Can you work these out from the model? Positions are in its coordinate system, mm. A direction names the side the tool comes from. Coordinates: 2 decimals unless noted, no trailing zeros. Order: outer loops, then holes, each group sorted by start corner. A loop starts at its lowest first (then second) coordinate and runs counter-clockwise, first axis right, second up. Notation, with made-up numbers: (50, -6.75) -> (77, -6.75) arc R29 ccw to (77, 20.25) -> close; hole circle Ø2 at (78.5, 27). An arc over 180 degrees is marked (long way). Answer as a JSON object with one key per item and string values. Group by question number.
(1) Which directions (+Z, -Z, +X, -X, +Y, -Y) give clear straight access to the entire face, cutting with the end or side of a thin tool? Please do faces 4 (the flat face through (31.5, -30, 0)), 5 (the flat face through (33, -29, 0)), 6 (the flat face through (-49, -59.5, 0)), 7 (the flat face through (-33, -29, 0)).
(2) I need wall thicknesses on line 1 (X direction, y = -59.1, z = 0); line 2 (X direction, y = -34.5, z = 6.5); line 3 (X direction, y = -58.45, z = 0). Which ranges of each line are inside material? Lowest first, please.
(3) I want a section at C-C, the plane z = 0. List the corners of the cut face in (x, y) for me, plus the area to 3 significant figures.
(4) For pin 1 (11.5 mm diameter, centred on x = 59, z = 0, fed in from +Y); pin 2 (20 mm diameter, centred on y = -29, z = 8.5, fed in from -X); pin 3 (20 mm diameter, centred on y = -35.5, z = -4, fed in from +X), each with a flat end and sliding along its axis, tell me the tip position at first contact or that it passes through.
(5) I want a section at D-D, the plane x = -43.5. List the corners of the cut face in (y, z) for me.
(6) I want a section at A-A, the plane x = 64.5. List the corners of the cut face in (y, z) for me.
(7) I want a section at B-B, the plane y = -17. List the corners of the cut face in (x, z) for me, plus the area to 3 significant figures.
(8) If we mould it in two halves opening along Z, with no side actions, what happens to faces 1 (the flat face through (70, -59, 18)), 2 (the cylindrical face through (61.57, -58.74, -0.65)), 3 (the flat face through (-50, -58, 0))? For each: pulls with the +Z half, pulls with the -Z half, needs draft (parallel to the pull), parting line crosses it, or undercut.
from build123d import *

# Parameters (mm, degrees)
SKETCH1_W          = 60
SKETCH1_H          = 40
BASE_FLANGE1_DEPTH = 1.5
EDGE_FLANGE1_DEPTH = 40
EDGE_FLANGE2_DEPTH = 40
CHAMFER1_SIZE      = 5
CUT_EXTRUDE1_REACH = 97.357
SKETCH10_R         = 2
SKETCH10_R_2       = 3


# Sheet-metal steps are written as plain solids
with BuildPart() as part:
    # Sketch1 → Base-Flange1 (new body)
    with BuildSketch(Plane(origin=(0, 0, 0), x_dir=(1, 0, 0), z_dir=(0, 1, 0))):
        Rectangle(SKETCH1_W, SKETCH1_H)
    extrude(amount=-BASE_FLANGE1_DEPTH)

    # Edge-Flange1 section (across the edge) → Edge-Flange1 (add)
    with BuildSketch(Plane(origin=(-31.5, -1.5, 20), x_dir=(1, 0, 0), z_dir=(0, 0, -1))):
        with BuildLine():
            Line((-1.5, 1.5), (-1.5, 55))
            Line((-1.5, 55), (0, 55))
            Line((0, 55), (0, 1.5))
            ThreePointArc((0, 1.5), (0.439339828, 0.439339828), (1.5, 0))
            Line((1.5, 0), (1.5, -1.5))
            ThreePointArc((1.5, -1.5), (-0.621320344, -0.621320344), (-1.5, 1.5))
        make_face()
    edge_flange1 = extrude(amount=EDGE_FLANGE1_DEPTH)

    # Edge-Flange2 section (across the edge) → Edge-Flange2 (add)
    with BuildSketch(Plane(origin=(-33, -58, -20), x_dir=(0, 1, 0), z_dir=(0, 0, 1))):
        with BuildLine():
            Line((-1.5, 1.5), (-1.5, 40))
            Line((-1.5, 40), (0, 40))
            Line((0, 40), (0, 1.5))
            ThreePointArc((0, 1.5), (0.439339828, 0.439339828), (1.5, 0))
            Line((1.5, 0), (1.5, -1.5))
            ThreePointArc((1.5, -1.5), (-0.621320344, -0.621320344), (-1.5, 1.5))
        make_face()
    edge_flange2 = extrude(amount=EDGE_FLANGE2_DEPTH)

    # Mirror1: Edge-Flange1, Edge-Flange2 across plane
    add(edge_flange1.mirror(Plane(origin=(0, 0, 0), x_dir=(0, 0, 1), z_dir=(1, 0, 0))))
    add(edge_flange2.mirror(Plane(origin=(0, 0, 0), x_dir=(0, 0, 1), z_dir=(1, 0, 0))))

    # Chamfer1
    chamfer1_edges = [part.edges().sort_by_distance(p)[0] for p in [
        (-73, -58.75, -20),
        (-73, -58.75, 20),
        (73, -58.75, 20),
        (73, -58.75, -20),
    ]]
    chamfer(chamfer1_edges, length=CHAMFER1_SIZE)

    # Sketch10 → Cut-Extrude1 (cut, up to next)
    with BuildSketch(Plane(origin=(0, -58, 0), x_dir=(1, 0, 0), z_dir=(0, 1, 0)), mode=Mode.PRIVATE) as cut_extrude1_sk1:
        with Locations(Location((-53, 0, 0), (0, 0, 270))):
            Circle(SKETCH10_R)
    cut_extrude1_tool1 = extrude(cut_extrude1_sk1.sketch, amount=-CUT_EXTRUDE1_REACH, mode=Mode.PRIVATE) & part.part
    # Sketch10 → Cut-Extrude1 (cut, up to next)
    with BuildSketch(Plane(origin=(0, -58, 0), x_dir=(1, 0, 0), z_dir=(0, 1, 0)), mode=Mode.PRIVATE) as cut_extrude1_sk2:
        with Locations(Location((64.5, 0, 0), (0, 0, 270))):
            Circle(SKETCH10_R_2)
    cut_extrude1_tool2 = extrude(cut_extrude1_sk2.sketch, amount=-CUT_EXTRUDE1_REACH, mode=Mode.PRIVATE) & part.part
    add(cut_extrude1_tool1.solids().sort_by_distance((-53, -58, 0))[0], mode=Mode.SUBTRACT)
    add(cut_extrude1_tool2.solids().sort_by_distance((64.5, -58, 0))[0], mode=Mode.SUBTRACT)


solid = part.part
Computed values:
{
 "1": {"face 4": "+Z, -Z, -Y", "face 5": "+Z, -Z, +X, +Y", "face 6": "+Z, -Z, +X, -X, -Y", "face 7": "+Z, -Z, -X, +Y"},
 "2": {"line 1": "x = -73 to -55, -51 to -33, 33 to 61.5, 67.5 to 73", "line 2": "x = -33 to -31.5, 31.5 to 33", "line 3": "x = -73 to -55, -51 to -32.22, 32.22 to 61.5, 67.5 to 73"},
 "3": {"outline": "(-73, -59.5) -> (-55, -59.5) -> (-55, -58) -> (-73, -58) -> close; (-51, -59.5) -> (-34.5, -59.5) arc R3 ccw to (-31.5, -56.5) -> (-31.5, -3) arc R1.5 cw to (-30, -1.5) -> (30, -1.5) arc R1.5 cw to (31.5, -3) -> (31.5, -56.5) arc R3 ccw to (34.5, -59.5) -> (61.5, -59.5) -> (61.5, -58) -> (34.5, -58) arc R1.5 cw to (33, -56.5) -> (33, -3) arc R3 ccw to (30, 0) -> (-30, 0) arc R3 ccw to (-33, -3) -> (-33, -56.5) arc R1.5 cw to (-34.5, -58) -> (-51, -58) -> close; (67.5, -59.5) -> (73, -59.5) -> (73, -58) -> (67.5, -58) -> close", "area": "372 mm2"},
 "4": {"pin 1": "stops at y = -58", "pin 2": "stops at x = -33", "pin 3": "stops at x = 33"},
 "5": {"outline": "(-59.5, -20) -> (-58, -20) -> (-58, 20) -> (-59.5, 20) -> close"},
 "6": {"outline": "(-59.5, -20) -> (-58, -20) -> (-58, -3) -> (-59.5, -3) -> close; (-59.5, 3) -> (-58, 3) -> (-58, 20) -> (-59.5, 20) -> close"},
 "7": {"outline": "(-33, -20) -> (-31.5, -20) -> (-31.5, 20) -> (-33, 20) -> close; (31.5, -20) -> (33, -20) -> (33, 20) -> (31.5, 20) -> close", "area": "120 mm2"},
 "8": {"face 1": "pulls with the +Z half", "face 2": "undercut", "face 3": "needs draft"}
}
